Design review of the part built by this model. Coordinates are the model's own, in mm. Coordinates: 2 decimals unless noted, no trailing zeros. Loops run counter-clockwise (first coordinate to the right, second up) from the corner with the lowest first, then second, coordinate; pieces in that order, holes last. Notation, with made-up numbers: (14, 17) -> (29, 17) arc R18 cw to (29, 44) -> close; hole circle Ø2 at (-39.75, 22). An arc over 180 degrees is marked (long way). Use a Markdown table: item, result. Add a question column.
Q1. Take a section at A-A on x = -16.5. Write out the cut boundary in (y, z).
Q2. Take a section at B-B on y = -1.1. Write out the cut boundary in (x, z).
Q3. Take a section at D-D on x = -23. Write out the cut boundary in (y, z).
Q4. Take a section at C-C on z = 26.5. Write out the cut boundary in (x, y).
Q5. For probe 1 along Z at (x, y) = (-17.5, -1); probe 2 along Z at (x, y) = (-16, -1.25); probe 3 along X at (y, z) = (-0.55, 35.5), list the stretches that pass through material, from the lowest coordinate up.
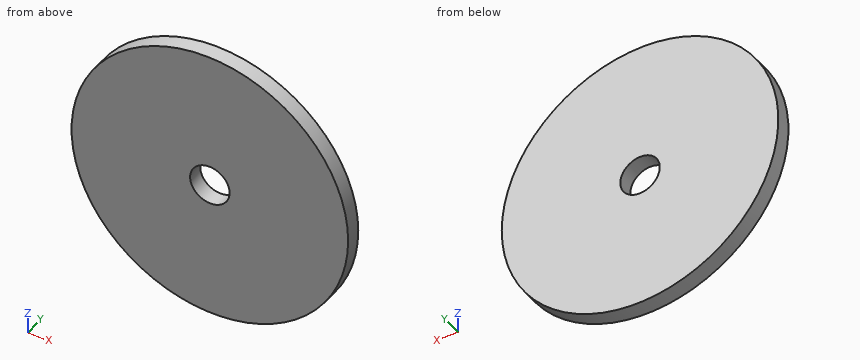
from build123d import *

# Parameters (mm, degrees)
F0_R     = 17.5
F1_DEPTH = 2.00000108
F2_R     = 2.5
F3_DEPTH = 6
F6_DEPTH = 8.00100108


# Not quite as in the source:
# - a feature of the source that left no trace in its solid (it failed there, or was rolled back) is left out


with BuildPart() as f1:
    # F0 (on Front) → F1 (new body)
    with BuildSketch(Plane.XZ):
        with Locations((-15.6701616943, 19.357258454)):
            Circle(F0_R)
    extrude(amount=F1_DEPTH)

    # F2 (on face) → F3 (join)
    with BuildSketch(Plane.XZ.offset(2.00000108)):
        with Locations((-15.6701616943, 19.357258454)):
            Circle(F2_R)
    extrude(amount=F3_DEPTH)

    # F6 (cut, through all): a face of the model
    f6_faces = [f1.faces().sort_by_distance(p)[0] for p in [
        (-15.6701616943, -8.00000108, 19.357258454),
    ]]
    extrude(f6_faces, amount=-F6_DEPTH, mode=Mode.SUBTRACT)


solid = f1.part
Answer list:
| question | item | result |
|---|---|---|
| 1 | outline | (-2, 1.88) -> (0, 1.88) -> (0, 17) -> (-2, 17) -> close; (-2, 21.72) -> (0, 21.72) -> (0, 36.84) -> (-2, 36.84) -> close |
| 2 | outline | circle Ø35 at (-15.67, 19.36); hole circle Ø5 at (-15.67, 19.36) |
| 3 | outline | (-2, 3.47) -> (0, 3.47) -> (0, 35.25) -> (-2, 35.25) -> close |
| 4 | outline | (-31.65, -2) -> (0.31, -2) -> (0.31, 0) -> (-31.65, 0) -> close |
| 5 | probe 1 | 1.95 to 17.65, 21.06 to 36.76 |
| 5 | probe 2 | 1.86 to 16.88, 21.84 to 36.85 |
| 5 | probe 3 | -22.43 to -8.91 |
